Design review of the part built by this model. Coordinates are the model's own, in mm. A direction names the side the tool comes from. Give positions to 0.01 mm unless a question says otherwise; leave off trailing zeros. Loops run counter-clockwise (first coordinate to the right, second up) from the corner with the lowest first, then second, coordinate; pieces in that order, holes last. Notation, with made-up numbers: (1, 13.25) - (50, 13.25) arc R31 cw to (50, 49.25) - close; hole circle Ø2 at (-27, 30.5). An arc over 180 degrees is marked (long way). Write each question's results on one line, items separated by ' | '.
from build123d import *

# Parameters (mm, degrees)
SKETCH1_W           = 31.001294418
SKETCH1_H           = 58.025746404
SKETCH1_R           = 1.3
BOSS_EXTRUDE1_DEPTH = 1.5
SKETCH2_W           = 6.985889014
SKETCH2_H           = 7.403537408
BOSS_EXTRUDE2_DEPTH = 2
SKETCH3_W           = 2.398141005
SKETCH3_H           = 46.294548095
SKETCH3_H_2         = 45.929613594
BOSS_EXTRUDE3_DEPTH = 10
SKETCH4_W           = 1.668272003
SKETCH4_H           = 20.801266543
BOSS_EXTRUDE4_DEPTH = 2


with BuildPart() as part:
    # Sketch1 → Boss-Extrude1 (new body)
    with BuildSketch(Plane(origin=(0, 0, 0), x_dir=(1, 0, 0), z_dir=(0, 1, 0))):
        with Locations((11.734043017, 25.235374996)):
            Rectangle(SKETCH1_W, SKETCH1_H)
        with Locations(Location((0, 0, 0), (0, 0, 270))):
            Circle(SKETCH1_R, mode=Mode.SUBTRACT)
        with Locations(Location((23.6, 0, 0), (0, 0, 270))):
            Circle(SKETCH1_R, mode=Mode.SUBTRACT)
        with Locations(Location((23.6, 51.15, 0), (0, 0, 270))):
            Circle(SKETCH1_R, mode=Mode.SUBTRACT)
        with Locations(Location((0, 51.15, 0), (0, 0, 270))):
            Circle(SKETCH1_R, mode=Mode.SUBTRACT)
    extrude(amount=BOSS_EXTRUDE1_DEPTH)

    # Sketch2 → Boss-Extrude2 (add)
    with BuildSketch(Plane(origin=(0, 0, 0), x_dir=(-1, 0, 0), z_dir=(0, -1, 0))):
        with Locations((-11.734043017, -0.075729502)):
            Rectangle(SKETCH2_W, SKETCH2_H)
    extrude(amount=BOSS_EXTRUDE2_DEPTH)

    # Sketch3 → Boss-Extrude3 (add)
    with BuildSketch(Plane(origin=(0, 1.5, 0), x_dir=(1, 0, 0), z_dir=(0, 1, 0))):
        with Locations((-0.152395008, 25.678509747)):
            Rectangle(SKETCH3_W, SKETCH3_H)
        with Locations((23.672614542, 25.860976997)):
            Rectangle(SKETCH3_W, SKETCH3_H_2)
    extrude(amount=BOSS_EXTRUDE3_DEPTH)

    # Sketch4 → Boss-Extrude4 (add)
    with BuildSketch(Plane(origin=(0, 0, 0), x_dir=(-1, 0, 0), z_dir=(0, -1, 0))):
        with Locations((-25.288753045, 21.742430489)):
            Rectangle(SKETCH4_W, SKETCH4_H)
    extrude(amount=BOSS_EXTRUDE4_DEPTH)


solid = part.part
(1) Wall thickness on line 1 along X through (y, z) = (1.1, -51.15); line 2 along Y through (x, z) = (23, -41.5); line 3 along X through (y, z) = (6.25, -14.5): over which ranges is each line inside the solid? List them lowest first. Write a range as from..to.
Answers below:
line 1: -3.77..-1.3, 1.3..22.3, 24.9..27.23 | line 2: 0..11.5 | line 3: -1.35..1.05, 22.47..24.87
(2) Take a section at C-C on z = -51.15. Give the boundary of the cut face in (x, y), plus the area to 3 significant figures.
Answers below:
outline: (-3.77, 0) - (-1.3, 0) - (-1.3, 1.5) - (-3.77, 1.5) - close; (1.3, 0) - (22.3, 0) - (22.3, 1.5) - (1.3, 1.5) - close; (24.9, 0) - (27.23, 0) - (27.23, 1.5) - (24.9, 1.5) - close | area: 38.7 mm2
(3) Take a section at A-A on y = 9. Give the boundary of the cut face in (x, z).
Answers below:
outline: (-1.35, -48.83) - (1.05, -48.83) - (1.05, -2.53) - (-1.35, -2.53) - close; (22.47, -48.83) - (24.87, -48.83) - (24.87, -2.9) - (22.47, -2.9) - close
(4) Draft analysis for pull direction Z (two halves, no side actions). For faces 5 (the flat face through (24, 6, -2.896)), 6 (the cylindrical face through (22.33, 0.74, -0.28)), 7 (the flat face through (26.123, -1, -22)), state which applies: pulls with the +Z half, pulls with the -Z half, needs draft (parallel to the pull), parting line crosses it, or undercut.
Answers below:
face 5: pulls with the +Z half | face 6: undercut | face 7: needs draft
(5) Take a section at D-D on z = 0. Give the boundary of the cut face in (x, y).
Answers below:
outline: (-3.77, 0) - (-1.3, 0) - (-1.3, 1.5) - (-3.77, 1.5) - close; (1.3, 0) - (8.24, 0) - (8.24, -2) - (15.23, -2) - (15.23, 0) - (22.3, 0) - (22.3, 1.5) - (1.3, 1.5) - close; (24.9, 0) - (27.23, 0) - (27.23, 1.5) - (24.9, 1.5) - close
(6) Insertion check: P1, Ø6, axis at x = 8, z = -35.5, coming from the +Y side; P2, Ø3, axis at y = 7, z = -19.5, coming from the -X side; P3, Ø8, axis at y = 6, z = -26.5, coming from the +X side; P4, Ø4, axis at x = 19, y = 6.5, coming from the -Z side. Each pin has a flat end and moves straight along its axis. Give the tip position at first contact, or say it passes through.
Answers below:
P1: y = 1.5 | P2: x = -1.35 | P3: x = 24.87 | P4: through
(7) Take a section at B-B on x = 23.6. Give the boundary of the cut face in (y, z), plus the area to 3 significant figures.
Answers below:
outline: (0, -54.25) - (1.5, -54.25) - (1.5, -52.45) - (0, -52.45) - close; (0, -49.85) - (1.5, -49.85) - (1.5, -48.83) - (11.5, -48.83) - (11.5, -2.9) - (1.5, -2.9) - (1.5, -1.3) - (0, -1.3) - close; (0, 1.3) - (1.5, 1.3) - (1.5, 3.78) - (0, 3.78) - close | area: 539 mm2
(8) Tool access review of faces 1 (the flat face through (12, -1, -3.626)), 2 (the flat face through (22.474, 6, -26)), 3 (the flat face through (25, -1, -11.342)), 4 (the flat face through (8.241, -1, 0)): name each direction out of +Z, -Z, +X, -X, +Y, -Y from which nothing blocks a thin tool from reaching the whole face with its end or side.
Answers below:
face 1: -Z, +X, -X, -Y | face 2: +Z, -Z, +Y | face 3: +Z, +X, -X, -Y | face 4: +Z, -Z, -X, -Y
